The model under review builds one solid part; all positions refer to its coordinate system, in mm. Coordinates: 2 decimals unless noted, no trailing zeros. Order: outer loops, then holes, each group sorted by start corner. A loop starts at its lowest first (then second) coordinate and runs counter-clockwise, first axis right, second up. Notation, with made-up numbers: (-26.75, -26) - (-22.75, -26) arc R22 ccw to (-22.75, -6) - close; hole circle Ø8 at (28.25, 84.25). An arc over 180 degrees is marked (long way). Answer in a Markdown table with one row per item.
```python
from build123d import *


with BuildPart() as part:
    # Sketch1 → Revolve1 (revolve)
    with BuildSketch(Plane.XY):
        Polygon((9.525, 0), (20.6375, 0), (20.6375, 5.55625), (18.0975, 5.55625), (18.0975, 5.30225), (12.065, 5.30225), (12.065, 5.55625), (9.525, 5.55625), align=None)
    revolve1 = revolve(axis=Axis((0, 28.620588043, 0), (0, -1, 0)))

    # Mirror1: Revolve1 across plane
    add(revolve1.mirror(Plane.ZX))


solid = part.part
```
Item 1: Clearance check with flat-ended pins moving along their axes: pin 1 Ø1 at (y, z) = (0, 8.5) entering from -X; pin 2 Ø2 at (x, y) = (1.5, -2) entering from +Z; pin 3 Ø21.5 at (x, z) = (0, 0) entering from -Y; pin 4 Ø11 at (x, z) = (-1, 0.5) entering from +Y. State where each tip first meets the part, or that it passes through.
Check values:
| item | result |
|---|---|
| pin 1 | x = -19.02 |
| pin 2 | z = 20.63 |
| pin 3 | y = -5.56 |
| pin 4 | through |
Item 2: Mouldability with a two-part tool opening along Z and no side actions: class faces 1 (the face through (4, -5.302, -12)), 2 (the face through (4, 5.302, -12)), 3 (the face through (9, -5.556, 4)) as +Z half, -Z half, draft (parallel to the pull), parting line (faces both ways), or undercut.
Check values:
| item | result |
|---|---|
| face 1 | undercut |
| face 2 | undercut |
| face 3 | draft |
Item 3: To check wall thickness, follow line 1 (Z direction, x = 0, y = -5.5) (1 decimal); line 2 (Z direction, x = 0, y = 2.25) (1 decimal); line 3 (Y direction, x = 12.5, z = 5.5). State the ranges of each line that lie inside material, in increasing order. Write a range as from..to.
Check values:
| item | result |
|---|---|
| line 1 | -20.6..-18.1, -12.1..-9.5, 9.5..12.1, 18.1..20.6 |
| line 2 | -20.6..-9.5, 9.5..20.6 |
| line 3 | -5.3..5.3 |
Item 4: We need section D-D, the plane z = -17.5. Write out the cut boundary in (x, y).
Check values:
| item | result |
|---|---|
| outline | (-10.94, -5.56) - (-4.61, -5.56) - (-4.61, -5.3) - (4.61, -5.3) - (4.61, -5.56) - (10.94, -5.56) - (10.94, 5.56) - (4.61, 5.56) - (4.61, 5.3) - (-4.61, 5.3) - (-4.61, 5.56) - (-10.94, 5.56) - close |
